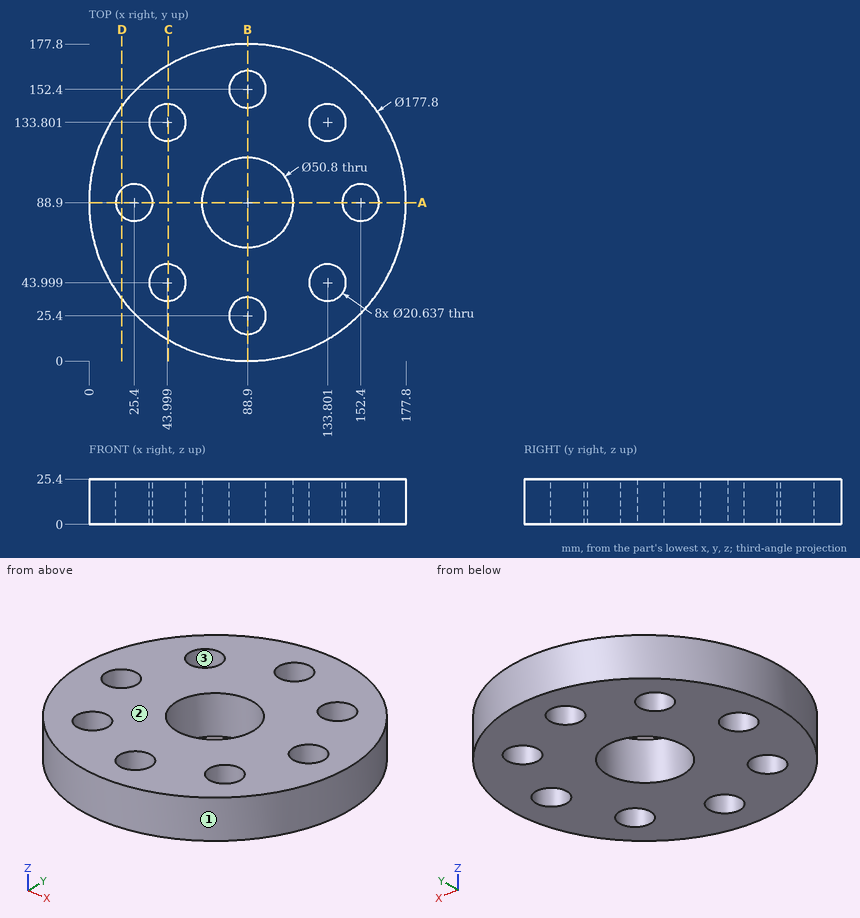
The figure shows three views and two pictorial views of one solid part (mm, origin at its lowest corner). Answer the questions. Coordinates: 2 decimals unless noted, no trailing zeros. Write each loop counter-clockwise with the first axis right and the second up, starting at its lowest first coordinate (ties: lowest second). Pieces come first, ordered by that corner, then holes.
1. The part is cut by section C-C, the plane x = 44.5. Write down the section's boundary in (y, z) (1 decimal), and give its area (3 significant figures).
Results list:
outline: (11.9, 0) - (33.7, 0) - (33.7, 25.4) - (11.9, 25.4) - close; (54.3, 0) - (123.5, 0) - (123.5, 25.4) - (54.3, 25.4) - close; (144.1, 0) - (165.9, 0) - (165.9, 25.4) - (144.1, 25.4) - close
area: 2,870 mm2
2. The part is cut by section D-D, the plane x = 18.5. Write down the section's boundary in (y, z), and give its area (3 significant figures).
Results list:
outline: (34.61, 0) - (81.23, 0) - (81.23, 25.4) - (34.61, 25.4) - close; (96.57, 0) - (143.19, 0) - (143.19, 25.4) - (96.57, 25.4) - close
area: 2,370 mm2
3. Flat-ended cylindrical pins translate along their axes: pin 1 (4 mm diameter, centred on x = 79, z = 2.5, fed in from +Y); pin 2 (5 mm diameter, centred on x = 79, z = 17, fed in from +Y); pin 3 (2 mm diameter, centred on x = 130.5, z = 20, fed in from +Y). Find the tip coordinate at first contact, or state that the pin passes through.
Results list:
pin 1: stops at y = 177.45
pin 2: stops at y = 177.49
pin 3: stops at y = 167.99
4. For a pull along X with two mould halves and no side action, classify the marked faces 1, 2 and 3 as +X half, -X half, draft (parallel to the pull), parting line (faces both ways), or undercut.
Results list:
face 1: parting line
face 2: draft
face 3: undercut
5. The part is cut by section A-A, the plane y = 88.9. Write down the section's boundary in (x, z), and give its area (3 significant figures).
Results list:
outline: (0, 0) - (15.08, 0) - (15.08, 25.4) - (0, 25.4) - close; (35.72, 0) - (63.5, 0) - (63.5, 25.4) - (35.72, 25.4) - close; (114.3, 0) - (142.08, 0) - (142.08, 25.4) - (114.3, 25.4) - close; (162.72, 0) - (177.8, 0) - (177.8, 25.4) - (162.72, 25.4) - close
area: 2,180 mm2
6. Consider line 1 along Y through (x, z) = (89.5, 22.75); line 2 along Y through (x, z) = (95.5, 4.25) (1 decimal); line 3 along X through (y, z) = (83, 12) (1 decimal). Determine where each line is inside the solid, lowest interval first.
Results list:
line 1: y = 0 to 15.1, 35.7 to 63.51, 114.29 to 142.1, 162.7 to 177.8
line 2: y = 0.2 to 17.5, 33.3 to 64.4, 113.4 to 144.5, 160.3 to 177.6
line 3: x = 0.2 to 16.9, 33.9 to 64.2, 113.6 to 143.9, 160.9 to 177.6
